Autodesk Inventor part; units mm, degrees
ref_plane "YZ Plane" through (0, 0, 0) normal (1, 0, 0) x (0, 1, 0)
ref_plane "XZ Plane" through (0, 0, 0) normal (0, 1, 0) x (-1, 0, 0)
ref_plane "XY Plane" through (0, 0, 0) normal (0, 0, 1) x (1, 0, 0)
sketch "Sketch1" plane through (0, 0, 0) normal (0, 1, 0) x (-1, 0, 0)
  line L0 (8.2489, 0) -> (4.1244, -7.1437)
  line L1 (4.1244, -7.1437) -> (-4.1244, -7.1437)
  line L2 (-4.1244, -7.1437) -> (-8.2489, 0)
  line L3 (-8.2489, 0) -> (-4.1244, 7.1437)
  line L4 (-4.1244, 7.1437) -> (4.1244, 7.1437)
  line L5 (4.1244, 7.1437) -> (8.2489, 0)
  point P0 (0, 0)
  point P1 (0, 0)
  dimension "d0" = 14.2875
extrude "Extrusion1" add sketch "Sketch1" along normal blind 8.3344
sketch "Sketch2" plane through (0, 8.3344, 0) normal (0, 1, 0) x (1, 0, 0)
  circle A0 centre (0, 0) radius 4.7625
  dimension "d3" = 9.525
hole "Hole1" at (0, 8.3344, 0) direction (0, -1, 0) diameter 7.7978 end through all
fillet "Fillet1" radius 1.524 6 edges at (0, 8.3344, 7.1437) (6.1867, 8.3344, 3.5719) (6.1867, 8.3344, -3.5719) (0, 8.3344, -7.1437) (-6.1867, 8.3344, -3.5719) (-6.1867, 8.3344, 3.5719)
properties part number "0nut_ss_375" material "Stainless Steel"
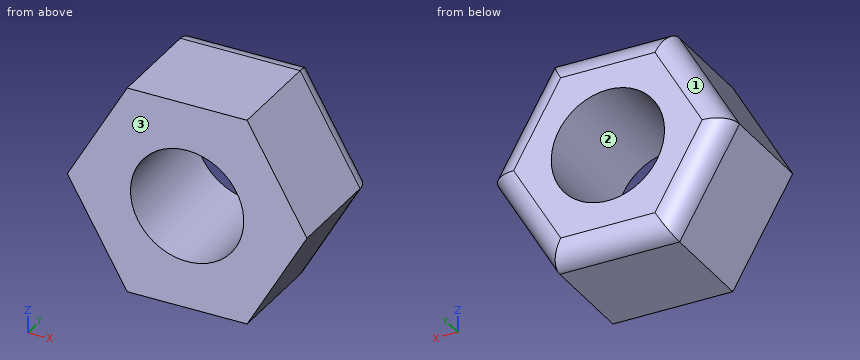
Can you work these out from the model? Positions are in its coordinate system, mm. Face numbers are marked on the shaded views. Round coordinates to 2 decimals unless told otherwise and drop trailing zeros. Loops run counter-clockwise (first coordinate to the right, second up) from the corner with the lowest first, then second, coordinate; pieces in that order, holes last. Notation, with made-up numbers: M -7,63.5 L 13,63.5 A11 ccw 13,83.5 Z; hole C 88.25,35.5 d5. An arc over 180 degrees is marked long. Write item = value, one per line. Start each with the question number.
(1) If we mould it in two halves opening along X, with no side actions, what happens to the marked faces 1, 2 and 3? For each: released by +X, released by -X, zero draft, split by the parting line, or undercut.
(2) I'm going to push flat-ended pins straight in: P1, Ø1, axis at y = 2.5, z = 1, coming from the +X side; P2, Ø5, axis at x = -6.5, z = -5.5, coming from the +Y side; P3, Ø2, axis at x = 6.5, y = 7, coming from the +Z side. Where does each tip first touch, or does it pass through?
(3) I need wall thicknesses on line 1 along Z through (x, y) = (2, 3.25); line 2 along Z through (x, y) = (0, 0.5); line 3 along X through (y, z) = (4.5, -1.25). Which ranges of each line are inside material? Lowest first, please.
(4) Suppose I cut it at C-C on y = 7.5. Write out the boundary of the cut face in (x, z), plus the area to 3 significant figures.
(5) Suppose I cut it at B-B on x = 0. Write out the boundary of the cut face in (y, z), plus the area to 3 significant figures.
(6) Suppose I cut it at A-A on y = 3.25. Write out the boundary of the cut face in (x, z).
(7) Suppose I cut it at D-D on x = -2.25. Write out the boundary of the cut face in (y, z).
Answer block:
q1.face_1 = released by -X
q1.face_2 = undercut
q1.face_3 = zero draft
q2.P1 = 7.96
q2.P2 = 8.31
q2.P3 = 4.75
q3.line_1 = -7.14 to -3.35, 3.35 to 7.14
q3.line_2 = -7.14 to -3.9, 3.9 to 7.14
q3.line_3 = -7.53 to -3.69, 3.69 to 7.53
q4.outline = M -8.06,0 L -4.03,-6.98 L 4.03,-6.98 L 8.06,0 L 4.03,6.98 L -4.03,6.98 Z; hole C 0,0 d7.8
q4.area = 121 mm²
q5.outline = M 0,-7.14 L 6.81,-7.14 A1.52 ccw 8.33,-5.62 L 8.33,-3.9 L 0,-3.9 Z; M 0,3.9 L 8.33,3.9 L 8.33,5.62 A1.52 ccw 6.81,7.14 L 0,7.14 Z
q5.area = 53.1 mm²
q6.outline = M -8.25,0 L -4.12,-7.14 L 4.12,-7.14 L 8.25,0 L 4.12,7.14 L -4.12,7.14 Z; hole C 0,0 d7.8
q7.outline = M 0,-7.14 L 6.81,-7.14 A1.52 ccw 8.33,-5.62 L 8.33,-3.18 L 0,-3.18 Z; M 0,3.18 L 8.33,3.18 L 8.33,5.62 A1.52 ccw 6.81,7.14 L 0,7.14 Z
